Geometry check sheet. Reference: the model listing, model coordinates, mm. Face numbers are marked on the shaded views. A direction names the side the tool comes from. Round coordinates to 2 decimals unless told otherwise and drop trailing zeros. Write each loop counter-clockwise with the first axis right and the second up, starting at its lowest first coordinate (ties: lowest second). Pieces come first, ordered by that corner, then holes.
Item 1: Scan lines: probe 1 along X at (y, z) = (8.25, 22.25); probe 2 along Y at (x, z) = (92, 5.75); probe 3 along Y at (x, z) = (92.5, 11). Record each from-to range of solid material in increasing order.
Item 2: Cross-section at D-D (x = 97). Enter the section's corners in (y, z), then the cut area to 3 significant figures.
Item 3: Cross-section at C-C (y = 20.75). Enter the section's corners in (x, z).
Item 4: Cross-section at B-B (z = 8.5). Enter the section's corners in (x, y).
Item 5: Depth check by flat-ended pin: P1, Ø1.3, axis at y = 1.5, z = 12, coming from the -X side; P2, Ø4, axis at x = 93.5, z = 15.5, coming from the +Y side; P3, Ø4, axis at x = 92, z = 7, coming from the +Y side. Enter the tip coordinate at first touch or a pass-through.
Item 6: Cross-section at A-A (z = 22.5). Enter the section's corners in (x, y), then the cut area to 3 significant figures.
Item 7: Access from +Z, -Z, +X, -X, +Y, -Y to the whole of each face (thin tool, end or side, straight path). Record for the marked faces 1 and 2.
from build123d import *

# Parameters (mm, degrees)
F1_DEPTH = 25.4
F2_R     = 3.81
F5_W     = 6.35
F5_H     = 2.54
F7_R     = 5.08
F8_R     = 5.08


with BuildPart() as f1:
    # F0 (on Top) → F1 (new body)
    with BuildSketch(Plane.XY):
        Polygon((104.9045048051, 0), (104.9045048051, 2.54), (104.9045048051, 22.86), (-23.3909259731, 2.54), (79.5045048051, 2.54), (79.5045048051, 0), align=None)
    extrude(amount=F1_DEPTH)

    # F2
    f2_edges = [f1.edges().sort_by_distance(p)[0] for p in [
        (104.904505, 0, 12.7),
    ]]
    fillet(f2_edges, radius=F2_R)

    # F5 (on offset) → F6 (revolve, cut)
    with BuildSketch(Plane(origin=(-4.938303697, 31.1792224467, 0), x_dir=(-0.9876883406, -0.156434465, 0), z_dir=(-0.156434465, 0.9876883406, 0))):
        with Locations((-89.706552875, 52.07)):
            Rectangle(F5_W, F5_H)
    revolve(axis=Axis((58.4876587146, 41.2249080053, 12.7), (-0.9876883406, -0.156434465, 0)), mode=Mode.SUBTRACT)

    # F7
    f7_edges = [f1.edges().sort_by_distance(p)[0] for p in [
        (89.283099, 9.733642, 25.4),
        (89.283099, 9.733642, 0),
    ]]
    fillet(f7_edges, radius=F7_R)

    # F8
    f8_edges = [f1.edges().sort_by_distance(p)[0] for p in [
        (-23.390926, 2.54, 12.7),
    ]]
    fillet(f8_edges, radius=F8_R)


solid = f1.part
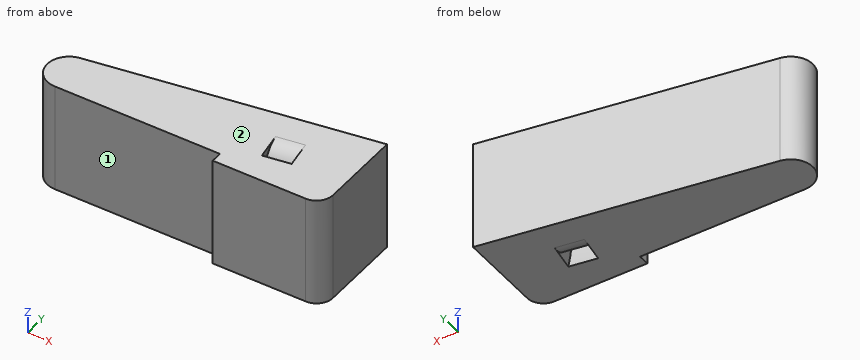
Resolved:
1. probe 1: x = 36.12 to 86.3, 92.73 to 104.9
1. probe 2: y = 0 to 5.99, 8.61 to 20.82
1. probe 3: y = 0 to 5.5, 8.08 to 20.9
2. outline: (0, 0) - (21.61, 0) - (21.61, 25.4) - (0, 25.4) - close
2. area: 549 mm2
3. outline: (91.58, 0) - (104.9, 0) - (104.9, 25.4) - (91.58, 25.4) - close
4. outline: (40.36, 12.64) arc R5.08 ccw to (41.16, 2.54) - (79.5, 2.54) - (79.5, 0) - (101.09, 0) arc R3.81 ccw to (104.9, 3.81) - (104.9, 22.86) - close; hole (86.45, 7.31) - (86.85, 4.79) - (93.12, 5.78) - (92.72, 8.31) - close
5. P1: stops at x = 79.5
5. P2: stops at y = 21.37
5. P3: stops at y = 21.13
6. outline: (40.36, 12.64) arc R5.08 ccw to (41.16, 2.54) - (79.5, 2.54) - (79.5, 0) - (101.09, 0) arc R3.81 ccw to (104.9, 3.81) - (104.9, 22.86) - close; hole (86.27, 8.45) - (86.7, 5.76) - (92.97, 6.75) - (92.54, 9.44) - close
6. area: 1,060 mm2
7. face 1: +Z, -Z, -X, -Y
7. face 2: +Z, +X, -X, +Y, -Y
